Can you work these out from the model? Positions are in its coordinate system, mm. A direction names the side the tool comes from. Round coordinates to 2 decimals unless told otherwise and drop trailing zeros. Write each loop counter-clockwise with the first axis right and the second up, starting at its lowest first coordinate (ties: lowest second). Pieces come first, ordered by that corner, then holes. Notation, with made-up numbers: (76, 5) -> (115, 5) arc R9 cw to (115, 22) -> close; hole circle Ø10 at (62, 2). An arc over 180 degrees is marked (long way). Write item = value, one per line. Start each with the question number.
1) Imagine slicing it at B-B, the plane z = 1.1. Please give me the cut outline in (x, y), then the cut area to 3 significant figures.
2) Thinking about a two-plate mould opening in X: for faces 1 (the face through (0, 4.74, 4)), 2 (the face through (-23, 4, 1)), 3 (the face through (-22.5, 0, 1.5)), which applies, +X half, -X half, draft (parallel to the pull), parting line (faces both ways), or undercut?
3) I'm going to push a flat-ended pin straight in: pin 1 (3.5 mm diameter, centred on x = 0, y = 0, fed in from +Z). Where does the tip first touch, or does it pass through?
4) For faces 4 (the face through (0, -4.74, 4)), 5 (the face through (0, 6, 4.56)), 6 (the face through (-16, -1.6, 1)), which set-ups out of +Z, -Z, +X, -X, +Y, -Y let a thin tool reach every point of the face, with its end or its side?
5) Imagine slicing it at C-C, the plane y = 0. Please give me the cut outline in (x, z), then the cut area to 3 significant figures.
6) Imagine slicing it at A-A, the plane x = -16. Please give me the cut outline in (y, z).
7) Imagine slicing it at D-D, the plane x = -20.5. Please give me the cut outline in (y, z), then the cut area to 3 significant figures.
8) If I drill on line 1 (Y direction, x = 0, z = 1.3); line 2 (X direction, y = -1, z = 2.2); line 3 (Z direction, x = 5, y = 0), over which ranges is the centre line in solid material (lowest first)?
from build123d import *

# Parameters (mm, degrees)
SKETCH_R        = 1.6
PAD_DEPTH       = 3
PAD001_DEPTH    = 20
SKETCH002_W     = 9.48
SKETCH002_H     = 9.48
POCKET_DEPTH    = 1.56
CHAMFER_SIZE    = 8
FILLET_R        = 3
SKETCH003_W     = 35
SKETCH003_H     = 3
POCKET001_DEPTH = 4.561
FILLET001_R     = 3


with BuildPart() as part:
    # Sketch → Pad (new body)
    with BuildSketch(Plane.XY):
        Polygon((-10, 10), (10, 10), (10, -10), (-10, -10), (-25, -10), (-25, 10), align=None)
        Circle(SKETCH_R, mode=Mode.SUBTRACT)
        with BuildLine():
            ThreePointArc((-20.9, 1.6), (-22.5, 0), (-20.9, -1.6))
            Line((-20.9, -1.6), (-11.6, -1.6))
            ThreePointArc((-11.6, -1.6), (-10, 0), (-11.6, 1.6))
            Line((-11.6, 1.6), (-20.9, 1.6))
        make_face(mode=Mode.SUBTRACT)
    extrude(amount=PAD_DEPTH)

    # Sketch001 (on Face3 of Pad) → Pad001 (join)
    with BuildSketch(Plane.XZ.offset(10)):
        Polygon((-4.74, 3), (4.74, 3), (2.94, 4.56), (-2.94, 4.56), align=None)
    extrude(amount=-PAD001_DEPTH)

    # Sketch002 (on Face18 of Pad001) → Pocket (cut)
    with BuildSketch(Plane.XY.offset(4.56)):
        Rectangle(SKETCH002_W, SKETCH002_H)
    extrude(amount=-POCKET_DEPTH, mode=Mode.SUBTRACT)

    # Chamfer
    chamfer_edges = [part.edges().sort_by_distance(p)[0] for p in [
        (-25, 10, 1.5),
        (-25, -10, 1.5),
    ]]
    chamfer(chamfer_edges, length=CHAMFER_SIZE)

    # Fillet
    fillet_edges = [part.edges().sort_by_distance(p)[0] for p in [
        (10, 10, 1.5),
        (10, -10, 1.5),
    ]]
    fillet(fillet_edges, radius=FILLET_R)

    # Sketch003 (on Face27 of Fillet) → Pocket001 (cut, through all)
    with BuildSketch(Plane.XY.offset(4.56)):
        with Locations((-7.5, 8.5)):
            Rectangle(SKETCH003_W, SKETCH003_H)
        with Locations((-7.5, -8.5)):
            Rectangle(SKETCH003_W, SKETCH003_H)
    extrude(amount=-POCKET001_DEPTH, mode=Mode.SUBTRACT)

    # Fillet001
    fillet001_edges = [part.edges().sort_by_distance(p)[0] for p in [
        (10, -7, 1.5),
        (10, 7, 1.5),
    ]]
    fillet(fillet001_edges, radius=FILLET001_R)


solid = part.part
Reported:
q1.outline = (-25, -2) -> (-20, -7) -> (7, -7) arc R3 ccw to (10, -4) -> (10, 4) arc R3 ccw to (7, 7) -> (-20, 7) -> (-25, 2) -> close; hole (-20.9, -1.6) -> (-11.6, -1.6) arc R1.6 ccw to (-11.6, 1.6) -> (-20.9, 1.6) arc R1.6 ccw to start; hole circle Ø3.2 at (0, 0)
q1.area = 415 mm²
q2.face_1 = draft
q2.face_2 = -X half
q2.face_3 = undercut
q3.pin_1 = 3
q4.face_4 = +Z, +X, -X
q4.face_5 = +Z, +X, -X, +Y, -Y
q4.face_6 = +Z, -Z
q5.outline = (-25, 0) -> (-22.5, 0) -> (-22.5, 3) -> (-25, 3) -> close; (-10, 0) -> (-1.6, 0) -> (-1.6, 3) -> (-10, 3) -> close; (1.6, 0) -> (10, 0) -> (10, 3) -> (1.6, 3) -> close
q5.area = 57.9 mm²
q6.outline = (-7, 0) -> (-1.6, 0) -> (-1.6, 3) -> (-7, 3) -> close; (1.6, 0) -> (7, 0) -> (7, 3) -> (1.6, 3) -> close
q7.outline = (-6.5, 0) -> (-1.6, 0) -> (-1.6, 3) -> (-6.5, 3) -> close; (1.6, 0) -> (6.5, 0) -> (6.5, 3) -> (1.6, 3) -> close
q7.area = 29.4 mm²
q8.line_1 = -7 to -1.6, 1.6 to 7
q8.line_2 = -25 to -22.15, -10.35 to -1.25, 1.25 to 10
q8.line_3 = 0 to 3
